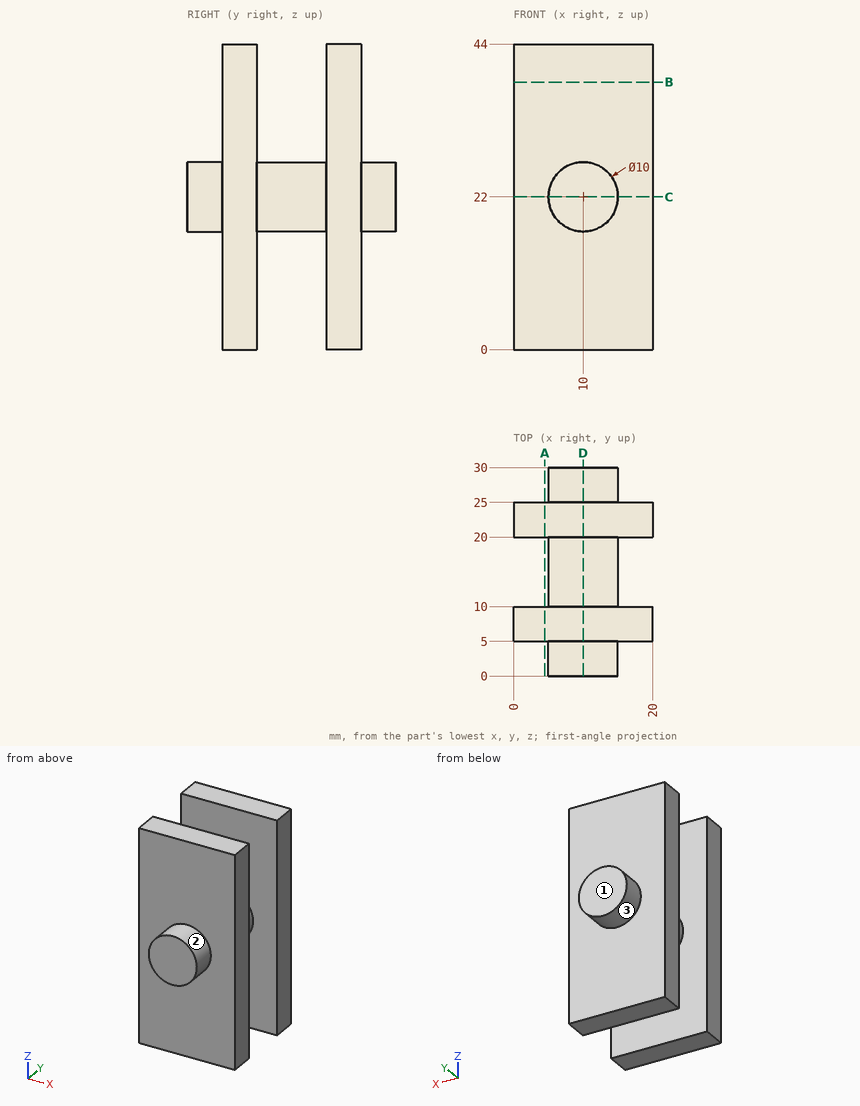
Here's the drawing with two shaded views (mm, measured from the low corner). I have some questions. A direction names the side the tool comes from. Give positions to 0.01 mm unless a question says otherwise; leave off trailing zeros. Write each loop counter-clockwise with the first axis right and the second up, starting at its lowest first coordinate (ties: lowest second). Pieces come first, ordered by that corner, then holes. Notation, with made-up numbers: (-23.5, 11.25) - (19.5, 11.25) arc R11 ccw to (19.5, 17.25) - close; hole circle Ø9 at (38, 54). An arc over 180 degrees is marked (long way). Write item = value, one per line. Start each with the question number.
1. For pin 1 (1.5 mm diameter, centred on x = 17, z = 11.5, fed in from +Y); pin 2 (6 mm diameter, centred on x = 11.5, z = 14, fed in from -Y), each with a flat end and sliding along its axis, tell me the tip position at first contact or that it passes through.
2. Imagine slicing it at C-C (z = 22). Please give me the cut outline in (x, y).
3. Please list where these lines run through material, in increasing order: line 1 (Y direction, x = 6.25, z = 16.5); line 2 (Z direction, x = 9.5, y = 10.25); line 3 (Z direction, x = 14, y = 10.75).
4. Imagine slicing it at B-B (z = 38.5). Please give me the cut outline in (x, y).
5. Imagine slicing it at D-D (x = 10). Please give me the cut outline in (y, z).
6. Imagine slicing it at A-A (x = 4.5). Please give me the cut outline in (y, z), and give its area (3 significant figures).
7. On a 3-axis mill with a long thin cutter (end or side, diameter ignored), from which of +Z, -Z, +X, -X, +Y, -Y can I reach the whole of each face in a straight line? I mean the marked faces 1, 2 and 3. Say none if no direction works.
Worked answers:
q1.pin_1 = 25
q1.pin_2 = 5
q2.outline = (0, 5) - (5, 5) - (5, 0) - (15, 0) - (15, 5) - (20, 5) - (20, 10) - (15, 10) - (15, 20) - (20, 20) - (20, 25) - (15, 25) - (15, 30) - (5, 30) - (5, 25) - (0, 25) - (0, 20) - (5, 20) - (5, 10) - (0, 10) - close
q3.line_1 = 5 to 10, 20 to 25
q3.line_2 = 17.03 to 26.97
q3.line_3 = 19 to 25
q4.outline = (0, 5) - (20, 5) - (20, 10) - (0, 10) - close; (0, 20) - (20, 20) - (20, 25) - (0, 25) - close
q5.outline = (0, 17) - (5, 17) - (5, 0) - (10, 0) - (10, 17) - (20, 17) - (20, 0) - (25, 0) - (25, 17) - (30, 17) - (30, 27) - (25, 27) - (25, 44) - (20, 44) - (20, 27) - (10, 27) - (10, 44) - (5, 44) - (5, 27) - (0, 27) - close
q6.outline = (5, 0) - (10, 0) - (10, 44) - (5, 44) - close; (20, 0) - (25, 0) - (25, 44) - (20, 44) - close
q6.area = 440 mm2
q7.face_1 = +Z, -Z, +X, -X, +Y
q7.face_2 = -Y
q7.face_3 = +Y
